Input: part model. Units: mm. Frame: model coordinates. A direction names the side the tool comes from. Give positions to 0.01 mm unless a question says otherwise; leave off trailing zeros. Order: outer loops, then holes, each group sorted by start corner. A loop starts at its lowest first (then second) coordinate and runs counter-clockwise, first axis right, second up. Notation, with made-up numbers: (40.5, 81.5) -> (95.5, 81.5) arc R21 ccw to (95.5, 102.5) -> close; hole circle Ø10 at (17.25, 68.5). An arc over 180 degrees is marked (long way). Use a Markdown table: item, result. Add a question column.
from build123d import *

# Parameters (mm, degrees)
ESQUISSE1_R      = 4
EXTRUSION1_DEPTH = 11.5
EXTRUSION2_DEPTH = 4.3
ESQUISSE3_R      = 6.35
EXTRUSION3_DEPTH = 14.2


with BuildPart() as part:
    # Esquisse1 → Extrusion1 (new body)
    with BuildSketch(Plane.XY):
        Circle(ESQUISSE1_R)
    extrude(amount=EXTRUSION1_DEPTH)

    # Esquisse2 → Extrusion2 (add)
    with BuildSketch(Plane.XY.offset(11.5)):
        Polygon((3.411005357, 8.429267018), (-5.594456694, 7.168650801), (-9.005462051, -1.260616217), (-3.411005357, -8.429267018), (5.594456694, -7.168650801), (9.005462051, 1.260616217), align=None)
    extrude(amount=EXTRUSION2_DEPTH)

    # Esquisse3 → Extrusion3 (add)
    with BuildSketch(Plane.XY.offset(15.8)):
        Circle(ESQUISSE3_R)
    extrude(amount=EXTRUSION3_DEPTH)

    # Esquisse4 → Révolution4 (revolve)
    with BuildSketch(Plane(origin=(0, 0, 0), x_dir=(1, 0, 0), z_dir=(0, 1, 0))):
        Polygon((0, -30), (0, -41.5), (-2.125, -41.5), (-2.25, -39), (-2.1, -39), (-2.25, -36), (-2.1, -36), (-2.25, -33), (-2.125, -33), (-2.25, -30), align=None)
    revolve(axis=Axis((0, 0, 18.076774383), (0, 0, 1)))


solid = part.part
Q1. Access query for faces 5 (the flat face through (-2, -4, 11.5)), 6 (the conical face through (0.472, 2.124, 37.479)), 7 (the flat face through (2, 6.3, 15.8)). Directions: +Z, -Z, +X, -X, +Y, -Y. A direction counts if a zero-diameter tool reaches every point of the face in a straight line with its end or side. Return the directions, or none.
Q2. Ray query, line 1 (Z direction, x = 2.5, y = -3.75); line 2 (Z direction, x = -7.5, y = -1.75); line 3 (Y direction, x = 4.25, z = 15.5). Return the intervals inside material, ascending.
Q3. Section query C-C (z = 19). Return loops of the section in (x, y).
Q4. Section query A-A (y = 0). Return loops of the section in (x, z) (3 decimals), plus the area to 3 significant figures.
Q5. Section query D-D (z = 3.5). Return loops of the section in (x, y), plus the area to 3 significant figures.
Q6. Draft query along Z for faces 1 (the flat face through (0, 0, 0)), 2 (the conical face through (-2.087, -0.657, 31.479)), 3 (the conical face through (0.472, 2.124, 34.479)), 4 (the flat face through (1.029, -7.808, 13.62)). Return one class per face: +Z half, -Z half, draft (parallel to the pull), parting line (faces both ways), or undercut.
Q7. Section query B-B (x = 0). Return loops of the section in (y, z) (3 decimals), plus the area to 3 significant figures.
Q8. First-contact query: pin 1 (1.5 mm diameter, centred on y = -3, z = 17.5, fed in from -X); pin 2 (3 mm diameter, centred on x = -5, y = -1, fed in from +Z); pin 3 (6 mm diameter, centred on x = -6, z = 26.5, fed in from -Y). Flat tips, straight axial feed; report the tip coordinate or a pass-through.
Solution:
| question | item | result |
|---|---|---|
| 1 | face 5 | -Z |
| 1 | face 6 | none |
| 1 | face 7 | +Z |
| 2 | line 1 | z = 11.5 to 30 |
| 2 | line 2 | z = 11.5 to 15.8 |
| 2 | line 3 | y = -7.36 to 7.35 |
| 3 | outline | circle Ø12.7 at (0, 0) |
| 4 | outline | (-8.495, 11.5) -> (-4, 11.5) -> (-4, 0) -> (4, 0) -> (4, 11.5) -> (8.495, 11.5) -> (8.495, 15.8) -> (6.35, 15.8) -> (6.35, 30) -> (2.25, 30) -> (2.125, 33) -> (2.25, 33) -> (2.1, 36) -> (2.25, 36) -> (2.1, 39) -> (2.25, 39) -> (2.125, 41.5) -> (-2.125, 41.5) -> (-2.25, 39) -> (-2.1, 39) -> (-2.25, 36) -> (-2.1, 36) -> (-2.25, 33) -> (-2.125, 33) -> (-2.25, 30) -> (-6.35, 30) -> (-6.35, 15.8) -> (-8.495, 15.8) -> close |
| 4 | area | 396 mm² |
| 5 | outline | circle Ø8 at (0, 0) |
| 5 | area | 50.3 mm² |
| 6 | face 1 | -Z half |
| 6 | face 2 | undercut |
| 6 | face 3 | undercut |
| 6 | face 4 | draft |
| 7 | outline | (-7.952, 11.5) -> (-4, 11.5) -> (-4, 0) -> (4, 0) -> (4, 11.5) -> (7.952, 11.5) -> (7.952, 15.8) -> (6.35, 15.8) -> (6.35, 30) -> (2.25, 30) -> (2.125, 33) -> (2.25, 33) -> (2.1, 36) -> (2.25, 36) -> (2.1, 39) -> (2.25, 39) -> (2.125, 41.5) -> (-2.125, 41.5) -> (-2.25, 39) -> (-2.1, 39) -> (-2.25, 36) -> (-2.1, 36) -> (-2.25, 33) -> (-2.125, 33) -> (-2.25, 30) -> (-6.35, 30) -> (-6.35, 15.8) -> (-7.952, 15.8) -> close |
| 7 | area | 391 mm² |
| 8 | pin 1 | stops at x = -5.94 |
| 8 | pin 2 | stops at z = 30 |
| 8 | pin 3 | stops at y = -5.6 |
